Here's how the part is built. I have some questions about the finished solid (model axes, mm). A direction names the side the tool comes from. Give positions to 0.01 mm unless a question says otherwise; leave off trailing zeros. Loops run counter-clockwise (first coordinate to the right, second up) from the corner with the lowest first, then second, coordinate; pieces in that order, holes last. Notation, with made-up numbers: (-22.5, 49.5) - (21.5, 49.5) arc R13 cw to (21.5, 66.5) - close; hole circle Ø11 at (13, 9). An arc over 180 degrees is marked (long way). Return JSON: item names as keys, results as strings. Group by question number.
(1) I need wall thicknesses on probe 1 along X at (y, z) = (60, 22); probe 2 along X at (y, z) = (7, 1); probe 3 along Y at (x, z) = (-29, 18). Which ranges of each line are inside material? Lowest first, please. Write a range as [from, to].
(2) If we mould it in two halves opening along Z, with no side actions, what happens to faces 1 (the cylindrical face through (11.18, 5.07, 19.71)), 2 (the flat face through (-27, 16, -36)), 3 (the flat face through (24.845, 69.444, 48.232))? For each: released by +Z, released by -Z, zero draft, split by the parting line, or undercut.
(3) If we section it at A-A (x = 10): State how many separate pieces and enclosed holes the cut face has, then the cut area to 3 significant figures.
(4) On a 3-axis mill with a long thin cutter (end or side, diameter ignored), from which of +Z, -Z, +X, -X, +Y, -Y can I reach the whole of each face in a straight line? I mean faces 4 (the cylindrical face through (-17, 50, 18)), 5 (the cylindrical face through (-8.82, 5.07, 19.71)), 6 (the cylindrical face through (-11.464, 106.07, -6.325)), 7 (the flat face through (-1.5, 82, 63)). Say none if no direction works.
(5) For P1, Ø3, axis at y = 81.5, z = -4.5, coming from the -X side; P2, Ø1.5, axis at x = -21.5, y = 68, coming from the +Z side; P3, Ø10, axis at y = 77.5, z = 56.5, coming from the -X side; P4, Ø3, axis at y = 67, z = -31, coming from the +X side, each with a flat end and sliding along its axis, tell me the tip position at first contact or that it passes through.
(6) If we section it at B-B (y = 103): Please give me the cut outline in (x, z).
```python
from build123d import *

# Parameters (mm, degrees)
SKETCH_1_W             = 67
SKETCH_1_H             = 62
EXTRUDE_1_DEPTH        = 10
SKETCH_3_W             = 14
SKETCH_3_H             = 20
EXTRUDE_2_DEPTH        = 12.5
SKETCH_4_W             = 10
SKETCH_4_H             = 65
EXTRUDE_3_DEPTH        = 67
SKETCH_5_W             = 67
SKETCH_5_H             = 44
EXTRUDE_4_DEPTH        = 8
EXTRUDE_5_DEPTH        = 20
CUT_EXTRUDE_START      = -6
CUT_EXTRUDE_1_DEPTH    = 8
EXTRUDE_6_DEPTH        = 6
SKETCH_9_R             = 3
CUT_EXTRUDE_2_DEPTH    = 23
SKETCH_10_W            = 24
SKETCH_10_H            = 23.8
EXTRUDE_7_DEPTH        = 8
SKETCH_12_W            = 14
SKETCH_12_H            = 20
EXTRUDE_8_DEPTH        = 11.5
SKETCH_13_R            = 0.95
CUT_EXTRUDE_4_DEPTH    = 8
SKETCH_14_W            = 8
SKETCH_14_H            = 6
EXTRUDE_9_DEPTH        = 11.8
SKETCH_15_R            = 0.95
CUT_EXTRUDE_5_DEPTH    = 11.8
SKETCH_16_W            = 3
SKETCH_16_H            = 6
EXTRUDE_10_DEPTH       = 12
FILLET_1_RADIUS        = 3
FILLET_1_LENGTH        = 3
SKETCH_17_R            = 1.75
CUT_EXTRUDE_6_DEPTH    = 7
SKETCH_18_R            = 3
EXTRUDE_11_DEPTH       = 36
FILLET_2_R             = 3
FILLET_2_OF_MIRROR_1_R = 3
SKETCH_20_R            = 1.75
CUT_EXTRUDE_7_DEPTH    = 35
SKETCH_21_W            = 15
SKETCH_21_H            = 55
CUT_EXTRUDE_8_DEPTH    = 35
SKETCH_24_R            = 1.75
CUT_EXTRUDE_11_DEPTH   = 18
SKETCH_25_R            = 1.5
CUT_EXTRUDE_12_DEPTH   = 10
FILLET_3_R             = 4
SKETCH_26_W            = 10.1
SKETCH_26_H            = 3.75
EXTRUDE_12_DEPTH       = 1
SKETCH_27_R            = 1.4
CUT_EXTRUDE_13_DEPTH   = 4


with BuildPart() as part:
    # 草图1 → 凸台-拉伸1 (new body)
    with BuildSketch(Plane(origin=(0, 0, 0), x_dir=(1, 0, 0), z_dir=(0, 1, 0))):
        Rectangle(SKETCH_1_W, SKETCH_1_H)
    extrude(amount=EXTRUDE_1_DEPTH)

    # 草图3 → 凸台-拉伸2 (add)
    with BuildSketch(Plane(origin=(0, 10, 0), x_dir=(1, 0, 0), z_dir=(0, 1, 0))):
        with Locations((-26.5, 26)):
            Rectangle(SKETCH_3_W, SKETCH_3_H)
    extrude(amount=EXTRUDE_2_DEPTH)

    # 草图4 → 凸台-拉伸3 (add)
    with BuildSketch(Plane.ZY.offset(33.5)):
        with Locations((-11, 42.5)):
            Rectangle(SKETCH_4_W, SKETCH_4_H)
    extrude(amount=-EXTRUDE_3_DEPTH)

    # 草图5 → 凸台-拉伸4 (add)
    with BuildSketch(Plane(origin=(0, 75, 0), x_dir=(1, 0, 0), z_dir=(0, 1, 0))):
        with Locations((0, -6)):
            Rectangle(SKETCH_5_W, SKETCH_5_H)
    extrude(amount=-EXTRUDE_4_DEPTH)

    # 草图6 → 凸台-拉伸5 (add)
    with BuildSketch(Plane(origin=(33.5, 0, 0), x_dir=(0, 0, -1), z_dir=(1, 0, 0))):
        with BuildLine():
            Line((-28, 60), (-28, 67))
            Line((-28, 67), (-8, 67))
            Line((-8, 67), (-8, 60))
            ThreePointArc((-8, 60), (-18, 50), (-28, 60))
        make_face()
    extrude_5 = extrude(amount=-EXTRUDE_5_DEPTH)

    # 草图7 → 切除-拉伸1 (cut)
    with BuildSketch(Plane(origin=(33.5, 0, 0), x_dir=(0, 0, -1), z_dir=(1, 0, 0)).offset(CUT_EXTRUDE_START)):
        with BuildLine():
            Line((-28, 60), (-28, 70.000230089))
            Line((-28, 70.000230089), (-8, 70.000230089))
            Line((-8, 70.000230089), (-8, 60))
            ThreePointArc((-8, 60), (-18, 50), (-28, 60))
        make_face()
    cut_extrude_1 = extrude(amount=-CUT_EXTRUDE_1_DEPTH, mode=Mode.SUBTRACT)

    # 草图8 → 凸台-拉伸6 (add)
    with BuildSketch(Plane(origin=(0, 75, 0), x_dir=(1, 0, 0), z_dir=(0, 1, 0))):
        Polygon((0, -68), (20, -68), (29.804375739, -28), (0, -28), align=None)
    extrude_6 = extrude(amount=-EXTRUDE_6_DEPTH)

    # 草图9 → 切除-拉伸2 (cut)
    with BuildSketch(Plane(origin=(33.5, 0, 0), x_dir=(0, 0, -1), z_dir=(1, 0, 0))):
        with Locations((-18, 60)):
            Circle(SKETCH_9_R)
    cut_extrude_2 = extrude(amount=-CUT_EXTRUDE_2_DEPTH, mode=Mode.SUBTRACT)

    # 草图10 → 凸台-拉伸7 (add)
    with BuildSketch(Plane(origin=(34.589358039, 0, 8.47817657), x_dir=(0.23806246083963745, 0, -0.9712498467124595), z_dir=(0.9712498467124595, 0, 0.23806246083963745))):
        Polygon((-49, 75), (-20, 75), (-20, 40.2), (-48, 40.2), (-54, 40.2), (-54, 75), align=None)
        with Locations((-37, 57.1)):
            Rectangle(SKETCH_10_W, SKETCH_10_H, mode=Mode.SUBTRACT)
    extrude_7 = extrude(amount=-EXTRUDE_7_DEPTH)

    # 草图12 → 凸台-拉伸8 (add)
    with BuildSketch(Plane(origin=(0, 75, 0), x_dir=(1, 0, 0), z_dir=(0, 1, 0))):
        with Locations((-26.5, 26)):
            Rectangle(SKETCH_12_W, SKETCH_12_H)
    extrude(amount=-EXTRUDE_8_DEPTH)

    # 草图13 → 切除-拉伸4 (cut)
    with BuildSketch(Plane(origin=(26.819359266, 0, 6.573676883), x_dir=(-0.23806246083963745, 0, 0.9712498467124595), z_dir=(-0.9712498467124595, 0, -0.23806246083963745))):
        with Locations((43.5, 70.95)):
            Circle(SKETCH_13_R)
        with Locations((31.5, 70.95)):
            Circle(SKETCH_13_R)
        with Locations((31.5, 43.25)):
            Circle(SKETCH_13_R)
        with Locations((43.5, 43.25)):
            Circle(SKETCH_13_R)
    cut_extrude_4 = extrude(amount=-CUT_EXTRUDE_4_DEPTH, mode=Mode.SUBTRACT)

    # 草图14 → 凸台-拉伸9 (add)
    with BuildSketch(Plane(origin=(0, 75, 0), x_dir=(1, 0, 0), z_dir=(0, 1, 0))):
        with Locations((7.7, -5)):
            Rectangle(SKETCH_14_W, SKETCH_14_H)
        with Locations((7.7, -34.8)):
            Rectangle(SKETCH_14_W, SKETCH_14_H)
    extrude(amount=EXTRUDE_9_DEPTH)

    # 草图15 → 切除-拉伸5 (cut)
    with BuildSketch(Plane.ZY.offset(-3.7)):
        with Locations((33.75, 81.5)):
            Circle(SKETCH_15_R)
        with Locations((6.05, 81.5)):
            Circle(SKETCH_15_R)
    extrude(amount=-CUT_EXTRUDE_5_DEPTH, mode=Mode.SUBTRACT)

    # 草图16 → 凸台-拉伸10 (add)
    with BuildSketch(Plane(origin=(0, 75, 0), x_dir=(1, 0, 0), z_dir=(0, 1, 0))):
        with Locations((0, -63)):
            Rectangle(SKETCH_16_W, SKETCH_16_H)
    extrude(amount=EXTRUDE_10_DEPTH)

    # 圆角1: full round fillet: the end face becomes a half cylinder, R = half its width
    fillet_1_face = Plane((0, 87, 63), x_dir=(1, 0, 0), z_dir=(0, 1, 0))  # on the end face: x along it, z out of the body
    fillet_1_slab = fillet_1_face.offset(-FILLET_1_RADIUS / 2) * Box(FILLET_1_LENGTH, 2 * FILLET_1_RADIUS, FILLET_1_RADIUS, mode=Mode.PRIVATE)  # the body's end, R deep
    fillet_1_round = Plane((0, 84, 63), x_dir=(0, 1, 0), z_dir=(1, 0, 0)) * Cylinder(FILLET_1_RADIUS, FILLET_1_LENGTH, mode=Mode.PRIVATE)  # its axis R under the face
    add(fillet_1_slab - fillet_1_round, mode=Mode.SUBTRACT)

    # 草图17 → 切除-拉伸6 (cut)
    with BuildSketch(Plane.ZY.offset(1.5)):
        with Locations((63, 84)):
            Circle(SKETCH_17_R)
    extrude(amount=-CUT_EXTRUDE_6_DEPTH, mode=Mode.SUBTRACT)

    # 草图18 → 凸台-拉伸11 (add)
    with BuildSketch(Plane(origin=(0, 75, 0), x_dir=(1, 0, 0), z_dir=(0, 1, 0))):
        with Locations(Location((10, 6, 0), (0, 0, 270))):
            Circle(SKETCH_18_R)
    extrude_11 = extrude(amount=EXTRUDE_11_DEPTH)

    # 圆角2
    fillet_2_edges = [part.edges().sort_by_distance(p)[0] for p in [
        (10, 75, -9),
    ]]
    fillet(fillet_2_edges, radius=FILLET_2_R)

    # 镜向1: 凸台-拉伸5, 切除-拉伸1, 凸台-拉伸6, 切除-拉伸2, 凸台-拉伸7, 切除-拉伸4, 凸台-拉伸11 across plane
    add(extrude_5.mirror(Plane(origin=(0, 0, 0), x_dir=(0, 0, 1), z_dir=(1, 0, 0))))
    add(cut_extrude_1.mirror(Plane(origin=(0, 0, 0), x_dir=(0, 0, 1), z_dir=(1, 0, 0))), mode=Mode.SUBTRACT)
    add(extrude_6.mirror(Plane(origin=(0, 0, 0), x_dir=(0, 0, 1), z_dir=(1, 0, 0))))
    add(cut_extrude_2.mirror(Plane(origin=(0, 0, 0), x_dir=(0, 0, 1), z_dir=(1, 0, 0))), mode=Mode.SUBTRACT)
    add(extrude_7.mirror(Plane(origin=(0, 0, 0), x_dir=(0, 0, 1), z_dir=(1, 0, 0))))
    add(cut_extrude_4.mirror(Plane(origin=(0, 0, 0), x_dir=(0, 0, 1), z_dir=(1, 0, 0))), mode=Mode.SUBTRACT)
    add(extrude_11.mirror(Plane(origin=(0, 0, 0), x_dir=(0, 0, 1), z_dir=(1, 0, 0))))

    # 圆角2 of 镜向1
    fillet_2_of_mirror_1_edges = [part.edges().sort_by_distance(p)[0] for p in [
        (-10, 75, -9),
    ]]
    fillet(fillet_2_of_mirror_1_edges, radius=FILLET_2_OF_MIRROR_1_R)

    # 草图20 → 切除-拉伸7 (cut)
    with BuildSketch(Plane.ZY.offset(33.5)):
        with Locations((-31, 67)):
            Circle(SKETCH_20_R)
        with Locations((-21, 67)):
            Circle(SKETCH_20_R)
        with Locations((-31, 19)):
            Circle(SKETCH_20_R)
        with Locations((-21, 19)):
            Circle(SKETCH_20_R)
    extrude(amount=-CUT_EXTRUDE_7_DEPTH, mode=Mode.SUBTRACT)

    # 草图21 → 切除-拉伸8 (cut)
    with BuildSketch(Plane(origin=(0, 0, -16), x_dir=(-1, 0, 0), z_dir=(0, 0, -1))):
        with Locations((0, 37.5)):
            Rectangle(SKETCH_21_W, SKETCH_21_H)
    extrude(amount=-CUT_EXTRUDE_8_DEPTH, mode=Mode.SUBTRACT)

    # 草图24 → 切除-拉伸11 (cut)
    with BuildSketch(Plane(origin=(0, 10, 0), x_dir=(1, 0, 0), z_dir=(0, 1, 0))):
        with Locations(Location((-10, -21, 0), (0, 0, 270))):
            Circle(SKETCH_24_R)
        with Locations(Location((10, -21, 0), (0, 0, 270))):
            Circle(SKETCH_24_R)
        with Locations(Location((-10, -1, 0), (0, 0, 270))):
            Circle(SKETCH_24_R)
        with Locations(Location((10, -1, 0), (0, 0, 270))):
            Circle(SKETCH_24_R)
    extrude(amount=-CUT_EXTRUDE_11_DEPTH, mode=Mode.SUBTRACT)

    # 草图25 → 切除-拉伸12 (cut)
    with BuildSketch(Plane(origin=(0, 111, 0), x_dir=(1, 0, 0), z_dir=(0, 1, 0))):
        with Locations(Location((10, 6, 0), (0, 0, 270))):
            Circle(SKETCH_25_R)
        with Locations(Location((-10, 6, 0), (0, 0, 270))):
            Circle(SKETCH_25_R)
    extrude(amount=-CUT_EXTRUDE_12_DEPTH, mode=Mode.SUBTRACT)

    # 圆角3
    fillet_3_edges = [part.edges().sort_by_distance(p)[0] for p in [
        (-1.5, 75, 63),
        (1.5, 75, 63),
    ]]
    fillet(fillet_3_edges, radius=FILLET_3_R)

    # 草图26 → 凸台-拉伸12 (add)
    with BuildSketch(Plane.XZ.offset(-69)):
        with Locations((0.05, 62.025)):
            Rectangle(SKETCH_26_W, SKETCH_26_H)
    extrude(amount=EXTRUDE_12_DEPTH)

    # 草图27 → 切除-拉伸13 (cut)
    with BuildSketch(Plane.XZ.offset(-68)):
        with Locations(Location((0, 62, 0), (0, 0, 270))):
            Circle(SKETCH_27_R)
    extrude(amount=-CUT_EXTRUDE_13_DEPTH, mode=Mode.SUBTRACT)


solid = part.part
```
Values:
{
 "1": {"probe 1": "[-33.5, -27.5], [-19.5, -13.5], [13.5, 19.5], [27.5, 33.5]", "probe 2": "[-33.5, -11.75], [-8.25, 8.25], [11.75, 33.5]", "probe 3": "[0, 10], [50, 57], [63, 75]"},
 "2": {"face 1": "undercut", "face 2": "released by -Z", "face 3": "released by +Z"},
 "3": {"separate pieces": "3", "enclosed holes": "2", "area": "2,040 mm2"},
 "4": {"face 4": "none", "face 5": "-Y", "face 6": "+Y", "face 7": "+Z, -Z, -X, +Y"},
 "5": {"P1": "x = -13", "P2": "z = 60.93", "P3": "x = -23.88", "P4": "through"},
 "6": {"outline": "circle Ø6 at (-10, -6); circle Ø6 at (10, -6); hole circle Ø3 at (-10, -6); hole circle Ø3 at (10, -6)"}
}
